Can you work these out from the model? Positions are in its coordinate system, mm. Coordinates: 2 decimals unless noted, no trailing zeros. Loops run counter-clockwise (first coordinate to the right, second up) from the corner with the lowest first, then second, coordinate; pieces in that order, holes last.
```python
from build123d import *

# Parameters (mm, degrees)
F1_DEPTH = 3


with BuildPart() as f1:
    # F0 (on Top) → F1 (new body)
    with BuildSketch(Plane.XY):
        with BuildLine():
            Line((95.5, 0), (90.5, 0))
            ThreePointArc((90.5, 0), (77.5, -13), (64.5, 0))
            Line((64.5, 0), (59.5, 0))
            ThreePointArc((59.5, 0), (46.5, -13), (33.5, 0))
            Line((33.5, 0), (28.5, 0))
            ThreePointArc((28.5, 0), (15.5, -13), (2.5, 0))
            Line((2.5, 0), (-2.5, 0))
            ThreePointArc((-2.5, 0), (-15.5, -13), (-28.5, 0))
            Line((-28.5, 0), (-33.5, 0))
            ThreePointArc((-33.5, 0), (-46.5, -13), (-59.5, 0))
            Line((-59.5, 0), (-64.5, 0))
            ThreePointArc((-64.5, 0), (-77.5, -13), (-90.5, 0))
            Line((-90.5, 0), (-95.5, 0))
            Line((-95.5, 0), (-95.5, -30))
            Line((-95.5, -30), (-63.5, -30))
            Line((-63.5, -30), (-63.5, -20.25))
            ThreePointArc((-63.5, -20.25), (-63.676777, -19.823223), (-63.25, -20))
            Line((-63.25, -20), (-60.85, -20))
            ThreePointArc((-60.85, -20), (-60.6, -19.75), (-60.35, -20))
            ThreePointArc((-60.35, -20), (-60.423223, -20.176777), (-60.6, -20.25))
            Line((-60.6, -20.25), (-60.6, -30))
            Line((-60.6, -30), (60.6, -30))
            Line((60.6, -30), (60.6, -20.25))
            ThreePointArc((60.6, -20.25), (60.423223, -19.823223), (60.85, -20))
            Line((60.85, -20), (63.25, -20))
            ThreePointArc((63.25, -20), (63.5, -19.75), (63.75, -20))
            ThreePointArc((63.75, -20), (63.676777, -20.176777), (63.5, -20.25))
            Line((63.5, -20.25), (63.5, -30))
            Line((63.5, -30), (95.5, -30))
            Line((95.5, -30), (95.5, 0))
        make_face()
    extrude(amount=F1_DEPTH)


solid = f1.part
```
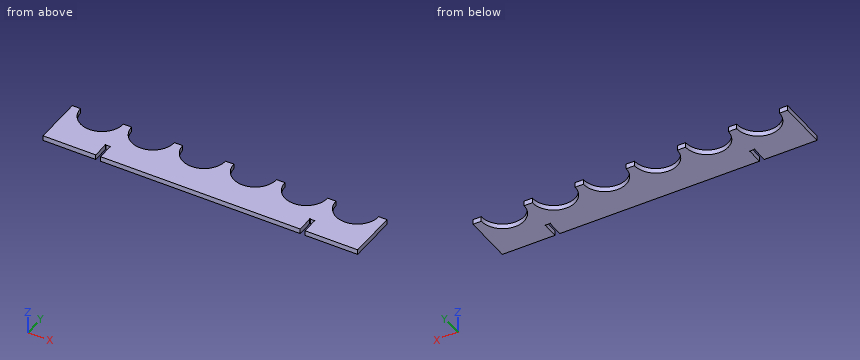
Item 1: Suppose I cut it at D-D, the plane x = 46.5. Please give me the cut outline in (y, z), plus the area to 3 significant figures.
Results are:
outline: (-30, 0) - (-13, 0) - (-13, 3) - (-30, 3) - close
area: 51.0 mm2
Item 2: I'm going to push a flat-ended pin straight in: P1, Ø0.7, axis at x = -62.5, z = 2, coming from the -Y side. Where does the tip first touch, or does it pass through?
Results are:
P1: stops at y = -20
Item 3: I need wall thicknesses on line 1 along X through (y, z) = (-22.5, 1.65); line 2 along Y through (x, z) = (-16, 0.7); line 3 along Y through (x, z) = (13.5, 2.1). Which ranges of each line are inside material? Lowest first, please.
Results are:
line 1: x = -95.5 to -63.5, -60.6 to 60.6, 63.5 to 95.5
line 2: y = -30 to -12.99
line 3: y = -30 to -12.85
Item 4: Suppose I cut it at A-A, the plane y = -26.5. Please give me the cut outline in (x, z), plus the area to 3 significant figures.
Results are:
outline: (-95.5, 0) - (-63.5, 0) - (-63.5, 3) - (-95.5, 3) - close; (-60.6, 0) - (60.6, 0) - (60.6, 3) - (-60.6, 3) - close; (63.5, 0) - (95.5, 0) - (95.5, 3) - (63.5, 3) - close
area: 556 mm2
Item 5: Suppose I cut it at B-B, the plane y = -10.25. Please give me the cut outline in (x, z).
Results are:
outline: (-95.5, 0) - (-85.5, 0) - (-85.5, 3) - (-95.5, 3) - close; (-69.5, 0) - (-54.5, 0) - (-54.5, 3) - (-69.5, 3) - close; (-38.5, 0) - (-23.5, 0) - (-23.5, 3) - (-38.5, 3) - close; (-7.5, 0) - (7.5, 0) - (7.5, 3) - (-7.5, 3) - close; (23.5, 0) - (38.5, 0) - (38.5, 3) - (23.5, 3) - close; (54.5, 0) - (69.5, 0) - (69.5, 3) - (54.5, 3) - close; (85.5, 0) - (95.5, 0) - (95.5, 3) - (85.5, 3) - close
